Can you work these out from the model? Positions are in its coordinate system, mm. A direction names the side the tool comes from. Coordinates: 2 decimals unless noted, no trailing zeros. Order: outer loops, then holes, each group sorted by start corner. A loop starts at its lowest first (then second) coordinate and runs counter-clockwise, first axis right, second up. Notation, with made-up numbers: (41.25, 20) -> (75.25, 20) arc R28 cw to (75.25, 38) -> close; hole circle Ø4 at (77, 5.5). An arc over 180 degrees is marked (long way). Return JSON: item names as keys, results as strings. Group by question number.
1) For faces 1 (the flat face through (11, 31, 2)), 2 (the flat face through (-20, 4.25, 4)), 3 (the flat face through (-19, 32, 5)), which set-ups out of +Z, -Z, +X, -X, +Y, -Y let a thin tool reach every point of the face, with its end or its side?
2) If we section it at D-D, the plane y = 11.5: Please give me the cut outline in (x, z), then the cut area to 3 significant figures.
3) If I drill on probe 1 along Y at (x, z) = (-35.65, 7.5); probe 2 along X at (y, z) = (33, 5.5); probe 3 along Z at (x, y) = (-30, 18), over which ranges is the centre line in solid material (lowest first)? Write a range as from..to.
4) If we section it at B-B, the plane y = 38: Please give me the cut outline in (x, z).
5) For pin 1 (2.5 mm diameter, centred on x = -38.5, z = 11.5, fed in from +Y); pin 2 (2 mm diameter, centred on y = 26, z = 4, fed in from -X); pin 3 (1.5 mm diameter, centred on y = 33.5, z = 2.5, fed in from +X); pin 4 (2 mm diameter, centred on x = -31, y = 15.5, fed in from -Z), each with a flat end and sliding along its axis, tell me the tip position at first contact or that it passes through.
6) Thinking about a two-plate mould opening in Z: for faces 4 (the flat face through (-36, 31, 15)), 5 (the cylindrical face through (-0.242, 56.247, 2.465)), 6 (the cylindrical face through (-38.524, 42.055, 6.169)), 7 (the cylindrical face through (-34.468, 44.133, 6.925)), which applies, +Z half, -Z half, draft (parallel to the pull), parting line (faces both ways), or undercut?
7) If we section it at A-A, the plane x = 0: Please give me the cut outline in (y, z).
from build123d import *

# Parameters (mm, degrees)
EXTRUDE_1_DEPTH      = 5
CUT_EXTRUDE_11_DEPTH = 5
EXTRUDE_2_DEPTH      = 10
CUT_EXTRUDE_12_REACH = 82.171
SKETCH_5_R           = 1.5
EXTRUDE_3_DEPTH      = 5
SKETCH_7_R           = 1.5
CUT_EXTRUDE_13_DEPTH = 5


with BuildPart() as part:
    # 草图2 → 凸台-拉伸1 (new body)
    with BuildSketch(Plane.XY):
        Polygon((12.999999835, 4.25), (-40.000000165, 4.25), (-40.003932239, 58.249999857), (12.996067761, 58.249999857), align=None)
    extrude(amount=EXTRUDE_1_DEPTH)

    # 草图3 → 切除-拉伸11 (cut)
    with BuildSketch(Plane.XY):
        with BuildLine():
            Line((-11, 17.25), (-11, 45.25))
            ThreePointArc((-11, 45.25), (0, 56.25), (11, 45.25))
            Line((11, 45.25), (11, 17.25))
            ThreePointArc((11, 17.25), (0, 6.25), (-11, 17.25))
        make_face()
    extrude(amount=CUT_EXTRUDE_11_DEPTH, mode=Mode.SUBTRACT)

    # 草图4 → 凸台-拉伸2 (add)
    with BuildSketch(Plane.XY.offset(5)):
        Polygon((-40.000000165, 4.25), (-37.000000165, 4.25), (-37.003932052, 58.247432028), (-40.003932052, 58.247432028), align=None)
    extrude(amount=EXTRUDE_2_DEPTH)

    # 草图5 → 切除-拉伸12 (cut, up to next)
    with BuildSketch(Plane(origin=(-39.999690484, -0.002912625, 0), x_dir=(0, 0, 1), z_dir=(-0.9999999973489005, -7.281619930679468e-05, 0)), mode=Mode.PRIVATE) as cut_extrude_12_sk1:
        with Locations(Location((7.5, 42.750344808, 0), (0, 0, 270))):
            Circle(SKETCH_5_R)
    cut_extrude_12_tool1 = extrude(cut_extrude_12_sk1.sketch, amount=-CUT_EXTRUDE_12_REACH, mode=Mode.PRIVATE) & part.part
    # 草图5 → 切除-拉伸12 (cut, up to next)
    with BuildSketch(Plane(origin=(-39.999690484, -0.002912625, 0), x_dir=(0, 0, 1), z_dir=(-0.9999999973489005, -7.281619930679468e-05, 0)), mode=Mode.PRIVATE) as cut_extrude_12_sk2:
        with Locations(Location((7.5, 22.750344808, 0), (0, 0, 270))):
            Circle(SKETCH_5_R)
    cut_extrude_12_tool2 = extrude(cut_extrude_12_sk2.sketch, amount=-CUT_EXTRUDE_12_REACH, mode=Mode.PRIVATE) & part.part
    add(cut_extrude_12_tool1.solids().sort_by_distance((-40.002803, 42.747432, 7.5))[0], mode=Mode.SUBTRACT)
    add(cut_extrude_12_tool2.solids().sort_by_distance((-40.001347, 22.747432, 7.5))[0], mode=Mode.SUBTRACT)

    # 草图6 → 凸台-拉伸3 (add)
    with BuildSketch(Plane(origin=(-36.9996905, -0.002694177, 0), x_dir=(0, 0, -1), z_dir=(0.9999999973489007, 7.281619931373636e-05, 0))):
        Polygon((-15, 58.25012636), (-5, 58.25012636), (-5, 4.249053378), (-15, 4.252694188), align=None)
    extrude(amount=EXTRUDE_3_DEPTH)

    # 草图7 → 切除-拉伸13 (cut)
    with BuildSketch(Plane(origin=(-31.999690513, -0.002330096, 0), x_dir=(0, 0, -1), z_dir=(0.9999999973489007, 7.281619931373636e-05, 0))):
        with Locations(Location((-7.5, 42.75012636, 0), (0, 0, 90))):
            Circle(SKETCH_7_R)
        with Locations(Location((-7.5, 22.75012636, 0), (0, 0, 90))):
            Circle(SKETCH_7_R)
    extrude(amount=-CUT_EXTRUDE_13_DEPTH, mode=Mode.SUBTRACT)


solid = part.part
Result sheet:
{
 "1": {"face 1": "+Z, -Z", "face 2": "+Z, -Z, +X, -X, -Y", "face 3": "+Z, +X, +Y, -Y"},
 "2": {"outline": "(-40, 0) -> (-9.38, 0) -> (-9.38, 5) -> (-32, 5) -> (-32, 15) -> (-40, 15) -> close; (9.38, 0) -> (13, 0) -> (13, 5) -> (9.38, 5) -> close", "area": "251 mm2"},
 "3": {"probe 1": "y = 4.25..21.25, 24.25..41.25, 44.25..58.25", "probe 2": "x = -40..-32", "probe 3": "z = 0..5"},
 "4": {"outline": "(-40, 0) -> (-11, 0) -> (-11, 5) -> (-32, 5) -> (-32, 15) -> (-40, 15) -> close; (11, 0) -> (13, 0) -> (13, 5) -> (11, 5) -> close"},
 "5": {"pin 1": "stops at y = 58.25", "pin 2": "stops at x = -40", "pin 3": "stops at x = 13", "pin 4": "stops at z = 0"},
 "6": {"face 4": "+Z half", "face 5": "draft", "face 6": "undercut", "face 7": "undercut"},
 "7": {"outline": "(4.25, 0) -> (6.25, 0) -> (6.25, 5) -> (4.25, 5) -> close; (56.25, 0) -> (58.25, 0) -> (58.25, 5) -> (56.25, 5) -> close"}
}
